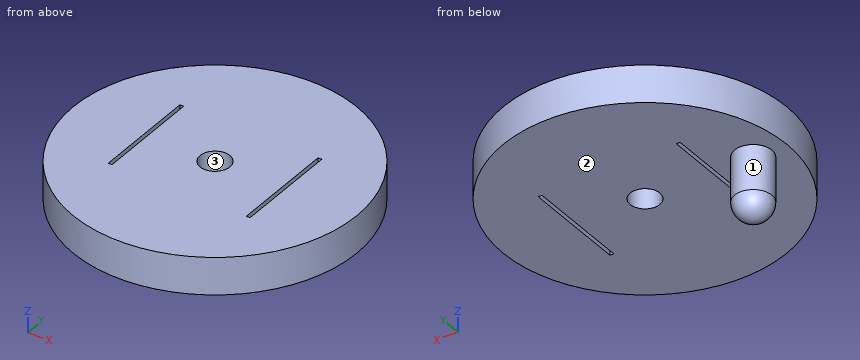
from build123d import *

# Parameters (mm, degrees)
SKETCH1_R           = 19
SKETCH1_R_2         = 2
SKETCH1_W           = 0.5
SKETCH1_H           = 14
BOSS_EXTRUDE1_DEPTH = 5


with BuildPart() as part:
    # Sketch1 → Boss-Extrude1 (new body)
    with BuildSketch(Plane.XY):
        Circle(SKETCH1_R)
        Circle(SKETCH1_R_2, mode=Mode.SUBTRACT)
        with Locations((-9.25, 0)):
            Rectangle(SKETCH1_W, SKETCH1_H, mode=Mode.SUBTRACT)
        with Locations((9.25, 0)):
            Rectangle(SKETCH1_W, SKETCH1_H, mode=Mode.SUBTRACT)
    extrude(amount=BOSS_EXTRUDE1_DEPTH)

    # Sketch3 → Revolve1 (revolve)
    with BuildSketch(Plane(origin=(0, 0, 0), x_dir=(1, 0, 0), z_dir=(0, 1, 0))):
        with BuildLine():
            Line((-17, 6), (-17, 0))
            Line((-17, 0), (-14.5, 0))
            Line((-14.5, 0), (-14.5, 8.5))
            ThreePointArc((-14.5, 8.5), (-16.267766953, 7.767766953), (-17, 6))
        make_face()
    revolve(axis=Axis((-14.5, 0, -6), (0, 0, 1)))


solid = part.part
Geometry: final body of the model. Coordinates: model frame, mm. Face numbers are marked on the shaded views. Give positions to 0.01 mm unless a question says otherwise; leave off trailing zeros. Write each loop counter-clockwise with the first axis right and the second up, starting at its lowest first coordinate (ties: lowest second). Pieces come first, ordered by that corner, then holes. Notation, with made-up numbers: (-33, 58.5) - (16, 58.5) arc R11 ccw to (16, 64.5) - close; hole circle Ø4 at (76, -10.75). An arc over 180 degrees is marked (long way). Return JSON: item names as keys, results as strings. Group by question number.
1) Line query: line 1 (Y direction, x = 0, z = 1.55); line 2 (Z direction, x = 13, y = -10.5); line 3 (X direction, y = 9, z = 2.75). Output: solid intervals per line, ascending.
2) Section B-B on x = 0. Return the cut outline in (y, z).
3) Section C-C on z = 2. Return the cut outline in (x, y).
4) Mould query, pull axis Y, two halves, no side actions, for the marked faces 1, 2 and 3. Classes: released by +Y, released by -Y, zero draft, split by the parting line, or undercut.
5) Section D-D on y = 5. Return the cut outline in (x, z), plus the area to 3 significant figures.
6) First-contact query: P1, Ø0.6, axis at x = -9, z = 1.5, coming from the +Y side; P2, Ø5, axis at x = 12.5, z = 0.5, coming from the -Y side; P3, Ø1.5, axis at x = -3.5, z = 0, coming from the +Y side. Flat tips, straight axial feed; report the tip coordinate or a pass-through.
7) Section A-A on y = 0. Return the cut outline in (x, z), plus the area to 3 significant figures.
Filled in:
{
 "1": {"line 1": "y = -19 to -2, 2 to 19", "line 2": "z = 0 to 5", "line 3": "x = -16.73 to 16.73"},
 "2": {"outline": "(-19, 0) - (-2, 0) - (-2, 5) - (-19, 5) - close; (2, 0) - (19, 0) - (19, 5) - (2, 5) - close"},
 "3": {"outline": "circle Ø38 at (0, 0); hole (-9.5, -7) - (-9, -7) - (-9, 7) - (-9.5, 7) - close; hole circle Ø4 at (0, 0); hole (9, -7) - (9.5, -7) - (9.5, 7) - (9, 7) - close"},
 "4": {"face 1": "split by the parting line", "face 2": "zero draft", "face 3": "undercut"},
 "5": {"outline": "(-18.33, 0) - (-9.5, 0) - (-9.5, 5) - (-18.33, 5) - close; (-9, 0) - (9, 0) - (9, 5) - (-9, 5) - close; (9.5, 0) - (18.33, 0) - (18.33, 5) - (9.5, 5) - close", "area": "178 mm^2"},
 "6": {"P1": "stops at y = 16.89", "P2": "stops at y = -16.16", "P3": "stops at y = 18.8"},
 "7": {"outline": "(-19, 0) - (-17, 0) - (-17, -6) arc R2.5 ccw to (-12, -6) - (-12, 0) - (-9.5, 0) - (-9.5, 5) - (-19, 5) - close; (-9, 0) - (-2, 0) - (-2, 5) - (-9, 5) - close; (2, 0) - (9, 0) - (9, 5) - (2, 5) - close; (9.5, 0) - (19, 0) - (19, 5) - (9.5, 5) - close", "area": "205 mm^2"}
}
